Read the model definition and answer for the solid it produces. Units are mm, in the model's axes. Round coordinates to 2 decimals unless told otherwise and drop trailing zeros. Put each result on its own line as item: value.
from build123d import *

# Parameters (mm, degrees)
F0_W     = 233.4336936474
F0_H     = 84.5690276474
F0_R     = 1.8721957215
F0_R_2   = 6.35
F1_DEPTH = 2.54


# Not quite as in the source:
# - a feature names something its author has since deleted; it is built from what else it names


with BuildPart() as f1:
    # F0 (on Front) → F1 (new body)
    with BuildSketch(Plane.XZ):
        with Locations((-11.6664916277, 61.8299962953)):
            Rectangle(F0_W, F0_H)
        with Locations((-104.3571985153, 29.2857964082)):
            Circle(F0_R, mode=Mode.SUBTRACT)
        with Locations((-112.2689694166, 32.5818173587)):
            Circle(F0_R, mode=Mode.SUBTRACT)
        with Locations((-115.3711608437, 39.9046507223)):
            Circle(F0_R, mode=Mode.SUBTRACT)
        with Locations((-104.3571985153, 39.9046507223)):
            Circle(F0_R_2, mode=Mode.SUBTRACT)
        with Locations((-96.2211242398, 32.574690507)):
            Circle(F0_R, mode=Mode.SUBTRACT)
        with Locations((-74.883861413, 32.3070631458)):
            Circle(F0_R, mode=Mode.SUBTRACT)
        with Locations((-93.3202734975, 39.9046507223)):
            Circle(F0_R, mode=Mode.SUBTRACT)
        with Locations((-77.9860528401, 39.6298965093)):
            Circle(F0_R, mode=Mode.SUBTRACT)
        with Locations((-66.9720905117, 29.0110421952)):
            Circle(F0_R, mode=Mode.SUBTRACT)
        with Locations((-28.7286259285, 28.620999728)):
            Circle(F0_R, mode=Mode.SUBTRACT)
        with Locations((-58.8360162362, 32.299936294)):
            Circle(F0_R, mode=Mode.SUBTRACT)
        with Locations((-66.9720905117, 39.6298965093)):
            Circle(F0_R_2, mode=Mode.SUBTRACT)
        with Locations((-55.9351654939, 39.6298965093)):
            Circle(F0_R, mode=Mode.SUBTRACT)
        with Locations((-36.6403968299, 31.9170206785)):
            Circle(F0_R, mode=Mode.SUBTRACT)
        with Locations((-20.5925516531, 31.9098938268)):
            Circle(F0_R, mode=Mode.SUBTRACT)
        with Locations((-39.742588257, 39.2398540421)):
            Circle(F0_R, mode=Mode.SUBTRACT)
        with Locations((-28.7286259285, 39.2398540421)):
            Circle(F0_R_2, mode=Mode.SUBTRACT)
        with Locations((-17.6917009107, 39.2398540421)):
            Circle(F0_R, mode=Mode.SUBTRACT)
        with Locations((-112.0281557075, 47.0351953909)):
            Circle(F0_R, mode=Mode.SUBTRACT)
        with Locations((-104.3571985153, 50.5235087617)):
            Circle(F0_R, mode=Mode.SUBTRACT)
        with Locations((-96.7241733432, 47.2419499663)):
            Circle(F0_R, mode=Mode.SUBTRACT)
        with Locations((-74.6430477039, 46.7604411779)):
            Circle(F0_R, mode=Mode.SUBTRACT)
        with Locations((-59.3390653396, 46.9671957533)):
            Circle(F0_R, mode=Mode.SUBTRACT)
        with Locations((-66.9720905117, 50.2487545487)):
            Circle(F0_R, mode=Mode.SUBTRACT)
        with Locations((-36.3995831207, 46.3703987107)):
            Circle(F0_R, mode=Mode.SUBTRACT)
        with Locations((-28.7286259285, 49.8587120814)):
            Circle(F0_R, mode=Mode.SUBTRACT)
        with Locations((-21.0956007565, 46.5771532861)):
            Circle(F0_R, mode=Mode.SUBTRACT)
        with Locations((6.8762816883, 29.1194615197)):
            Circle(F0_R, mode=Mode.SUBTRACT)
        with Locations((44.2613896919, 28.8447073068)):
            Circle(F0_R, mode=Mode.SUBTRACT)
        with Locations((-1.035489213, 32.4154824703)):
            Circle(F0_R, mode=Mode.SUBTRACT)
        with Locations((15.0123559638, 32.4083556185)):
            Circle(F0_R, mode=Mode.SUBTRACT)
        with Locations((-4.1376806401, 39.7383158338)):
            Circle(F0_R, mode=Mode.SUBTRACT)
        with Locations((6.8762816883, 39.7383158338)):
            Circle(F0_R_2, mode=Mode.SUBTRACT)
        with Locations((36.3496187906, 32.1407282573)):
            Circle(F0_R, mode=Mode.SUBTRACT)
        with Locations((17.9132067062, 39.7383158338)):
            Circle(F0_R, mode=Mode.SUBTRACT)
        with Locations((33.2474273635, 39.4635616208)):
            Circle(F0_R, mode=Mode.SUBTRACT)
        with Locations((44.2613896919, 39.4635616208)):
            Circle(F0_R_2, mode=Mode.SUBTRACT)
        with Locations((82.5048542751, 28.4546648395)):
            Circle(F0_R, mode=Mode.SUBTRACT)
        with Locations((52.3974639674, 32.1336014056)):
            Circle(F0_R, mode=Mode.SUBTRACT)
        with Locations((74.5930833738, 31.7506857901)):
            Circle(F0_R, mode=Mode.SUBTRACT)
        with Locations((55.2983147098, 39.4635616208)):
            Circle(F0_R, mode=Mode.SUBTRACT)
        with Locations((71.4908919467, 39.0735191536)):
            Circle(F0_R, mode=Mode.SUBTRACT)
        with Locations((90.6409285506, 31.7435589383)):
            Circle(F0_R, mode=Mode.SUBTRACT)
        with Locations((82.5048542751, 39.0735191536)):
            Circle(F0_R_2, mode=Mode.SUBTRACT)
        with Locations((93.5417792929, 39.0735191536)):
            Circle(F0_R, mode=Mode.SUBTRACT)
        with Locations((-0.7946755039, 46.8688605024)):
            Circle(F0_R, mode=Mode.SUBTRACT)
        with Locations((14.5093068604, 47.0756150778)):
            Circle(F0_R, mode=Mode.SUBTRACT)
        with Locations((6.8762816883, 50.3571738732)):
            Circle(F0_R, mode=Mode.SUBTRACT)
        with Locations((36.5904324997, 46.5941062895)):
            Circle(F0_R, mode=Mode.SUBTRACT)
        with Locations((44.2613896919, 50.0824196602)):
            Circle(F0_R, mode=Mode.SUBTRACT)
        with Locations((51.894414864, 46.8008608649)):
            Circle(F0_R, mode=Mode.SUBTRACT)
        with Locations((74.8338970829, 46.2040638222)):
            Circle(F0_R, mode=Mode.SUBTRACT)
        with Locations((90.1378794472, 46.4108183976)):
            Circle(F0_R, mode=Mode.SUBTRACT)
        with Locations((82.5048542751, 49.692377193)):
            Circle(F0_R, mode=Mode.SUBTRACT)
        with Locations((-103.9882795885, 73.0159394443)):
            Circle(F0_R, mode=Mode.SUBTRACT)
        with Locations((-111.9000504898, 76.3119603949)):
            Circle(F0_R, mode=Mode.SUBTRACT)
        with Locations((-95.852205313, 76.3048335431)):
            Circle(F0_R, mode=Mode.SUBTRACT)
        with Locations((-74.5149424862, 76.0372061819)):
            Circle(F0_R, mode=Mode.SUBTRACT)
        with Locations((-28.3597070018, 72.3511427641)):
            Circle(F0_R, mode=Mode.SUBTRACT)
        with Locations((-66.6031715849, 72.7411852313)):
            Circle(F0_R, mode=Mode.SUBTRACT)
        with Locations((-58.4670973094, 76.0300793301)):
            Circle(F0_R, mode=Mode.SUBTRACT)
        with Locations((-36.2714779031, 75.6471637146)):
            Circle(F0_R, mode=Mode.SUBTRACT)
        with Locations((-20.2236327263, 75.6400368629)):
            Circle(F0_R, mode=Mode.SUBTRACT)
        with Locations((-39.3736693302, 82.9699970782)):
            Circle(F0_R, mode=Mode.SUBTRACT)
        with Locations((-28.3597070018, 82.9699970782)):
            Circle(F0_R_2, mode=Mode.SUBTRACT)
        with Locations((-17.3227819839, 82.9699970782)):
            Circle(F0_R, mode=Mode.SUBTRACT)
        with Locations((-115.002241917, 83.6347937584)):
            Circle(F0_R, mode=Mode.SUBTRACT)
        with Locations((-103.9882795885, 83.6347937584)):
            Circle(F0_R_2, mode=Mode.SUBTRACT)
        with Locations((-111.6592367807, 90.765338427)):
            Circle(F0_R, mode=Mode.SUBTRACT)
        with Locations((-92.9513545707, 83.6347937584)):
            Circle(F0_R, mode=Mode.SUBTRACT)
        with Locations((-77.6171339134, 83.3600395454)):
            Circle(F0_R, mode=Mode.SUBTRACT)
        with Locations((-96.3552544164, 90.9720930024)):
            Circle(F0_R, mode=Mode.SUBTRACT)
        with Locations((-74.2741287771, 90.490584214)):
            Circle(F0_R, mode=Mode.SUBTRACT)
        with Locations((-103.9882795885, 94.2536517978)):
            Circle(F0_R, mode=Mode.SUBTRACT)
        with Locations((-66.6031715849, 83.3600395454)):
            Circle(F0_R_2, mode=Mode.SUBTRACT)
        with Locations((-55.5662465671, 83.3600395454)):
            Circle(F0_R, mode=Mode.SUBTRACT)
        with Locations((-58.9701464129, 90.6973387894)):
            Circle(F0_R, mode=Mode.SUBTRACT)
        with Locations((-36.030664194, 90.1005417468)):
            Circle(F0_R, mode=Mode.SUBTRACT)
        with Locations((-20.7266818297, 90.3072963222)):
            Circle(F0_R, mode=Mode.SUBTRACT)
        with Locations((-66.6031715849, 93.9788975848)):
            Circle(F0_R, mode=Mode.SUBTRACT)
        with Locations((-28.3597070018, 93.5888551176)):
            Circle(F0_R, mode=Mode.SUBTRACT)
        with Locations((-0.6665702862, 76.1456255064)):
            Circle(F0_R, mode=Mode.SUBTRACT)
        with Locations((7.2452006151, 72.8496045558)):
            Circle(F0_R, mode=Mode.SUBTRACT)
        with Locations((15.3812748906, 76.1384986547)):
            Circle(F0_R, mode=Mode.SUBTRACT)
        with Locations((44.6303086187, 72.5748503429)):
            Circle(F0_R, mode=Mode.SUBTRACT)
        with Locations((36.7185377174, 75.8708712934)):
            Circle(F0_R, mode=Mode.SUBTRACT)
        with Locations((82.8737732019, 72.1848078756)):
            Circle(F0_R, mode=Mode.SUBTRACT)
        with Locations((52.7663828942, 75.8637444417)):
            Circle(F0_R, mode=Mode.SUBTRACT)
        with Locations((74.9620023005, 75.4808288262)):
            Circle(F0_R, mode=Mode.SUBTRACT)
        with Locations((71.8598108734, 82.8036621897)):
            Circle(F0_R, mode=Mode.SUBTRACT)
        with Locations((91.0098474773, 75.4737019744)):
            Circle(F0_R, mode=Mode.SUBTRACT)
        with Locations((82.8737732019, 82.8036621897)):
            Circle(F0_R_2, mode=Mode.SUBTRACT)
        with Locations((93.9106982197, 82.8036621897)):
            Circle(F0_R, mode=Mode.SUBTRACT)
        with Locations((-3.7687617133, 83.4684588699)):
            Circle(F0_R, mode=Mode.SUBTRACT)
        with Locations((7.2452006151, 83.4684588699)):
            Circle(F0_R_2, mode=Mode.SUBTRACT)
        with Locations((-0.4257565771, 90.5990035386)):
            Circle(F0_R, mode=Mode.SUBTRACT)
        with Locations((14.8782257872, 90.805758114)):
            Circle(F0_R, mode=Mode.SUBTRACT)
        with Locations((18.2821256329, 83.4684588699)):
            Circle(F0_R, mode=Mode.SUBTRACT)
        with Locations((33.6163462903, 83.193704657)):
            Circle(F0_R, mode=Mode.SUBTRACT)
        with Locations((44.6303086187, 83.193704657)):
            Circle(F0_R_2, mode=Mode.SUBTRACT)
        with Locations((36.9593514265, 90.3242493256)):
            Circle(F0_R, mode=Mode.SUBTRACT)
        with Locations((7.2452006151, 94.0873169093)):
            Circle(F0_R, mode=Mode.SUBTRACT)
        with Locations((44.6303086187, 93.8125626963)):
            Circle(F0_R, mode=Mode.SUBTRACT)
        with Locations((55.6672336365, 83.193704657)):
            Circle(F0_R, mode=Mode.SUBTRACT)
        with Locations((52.2633337908, 90.531003901)):
            Circle(F0_R, mode=Mode.SUBTRACT)
        with Locations((75.2028160097, 89.9342068583)):
            Circle(F0_R, mode=Mode.SUBTRACT)
        with Locations((82.8737732019, 93.4225202291)):
            Circle(F0_R, mode=Mode.SUBTRACT)
        with Locations((90.5067983739, 90.1409614337)):
            Circle(F0_R, mode=Mode.SUBTRACT)
    extrude(amount=F1_DEPTH)


solid = f1.part
Item 1: The part is cut by section A-A (y = -2.05). State how many separate pieces and enclosed holes the cut face has, then the cut area to 3 significant figures.
Derived:
separate pieces: 1
enclosed holes: 108
area: 17,200 mm^2
Item 2: Find the intervals of material crossed by line 1 along Z through (x, y) = (47.5, -0.65); line 2 along Z through (x, y) = (-17, -1.95); line 3 along Z through (x, y) = (-74, -2.2), in increasing order.
Derived:
line 1: z = 19.55 to 34, 44.93 to 77.53, 88.86 to 104.11
line 2: z = 19.55 to 37.5, 40.98 to 81.13, 84.81 to 104.11
line 3: z = 19.55 to 30.66, 33.96 to 45, 48.52 to 74.24, 77.84 to 88.64, 92.34 to 104.11
Item 3: A flat-ended cylindrical pin translates along its axis: pin 1 Ø3 at (x, z) = (-0.43, 90.6) entering from -Y. Find the tip coordinate at first contact, or state that the pin passes through.
Derived:
pin 1: passes through
